Could you check a few things on this model? Use its own coordinates, in mm. Face numbers are marked on the shaded views. A direction names the side the tool comes from. Coordinates: 2 decimals unless noted, no trailing zeros. Loops run counter-clockwise (first coordinate to the right, second up) from the corner with the lowest first, then second, coordinate; pieces in that order, holes last. Notation, with made-up numbers: (57, 64) -> (90, 64) arc R21 cw to (90, 85) -> close; hole circle Ø10 at (57, -12). An arc over 180 degrees is marked (long way). One line per question, with ' | ' between items.
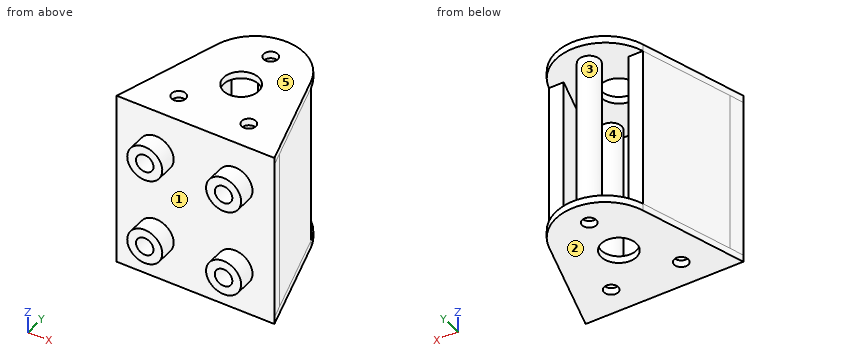
from build123d import *

# Parameters (mm, degrees)
SKETCH1_R           = 5
SKETCH1_R_2         = 2
BOSS_EXTRUDE1_DEPTH = 2
SKETCH2_R           = 2
SKETCH2_R_2         = 5
BOSS_EXTRUDE2_DEPTH = 2
SKETCH3_R           = 3
SKETCH3_R_2         = 2.5
BOSS_EXTRUDE3_DEPTH = 46
BOSS_EXTRUDE4_DEPTH = 46
BOSS_EXTRUDE5_DEPTH = 46
SKETCH8_R           = 5
SKETCH8_R_2         = 2.5
BOSS_EXTRUDE6_DEPTH = 5


with BuildPart() as part:
    # Sketch1 → Boss-Extrude1 (new body)
    with BuildSketch(Plane.XY):
        with BuildLine():
            Line((-22.5, 0), (22.5, 0))
            Line((22.5, 0), (13.399264765, 30.057056046))
            ThreePointArc((13.399264765, 30.057056046), (0, 40), (-13.399264765, 30.057056046))
            Line((-13.399264765, 30.057056046), (-22.5, 0))
        make_face()
        with Locations((0, 20)):
            Circle(SKETCH1_R, mode=Mode.SUBTRACT)
        with Locations((0, 33)):
            Circle(SKETCH1_R_2, mode=Mode.SUBTRACT)
        with Locations((10, 8)):
            Circle(SKETCH1_R_2, mode=Mode.SUBTRACT)
        with Locations((-10, 8)):
            Circle(SKETCH1_R_2, mode=Mode.SUBTRACT)
    extrude(amount=BOSS_EXTRUDE1_DEPTH)



with BuildPart() as body_2:
    # Sketch2 → Boss-Extrude2 (new body)
    with BuildSketch(Plane(origin=(0, 0, 50), x_dir=(-1, 0, 0), z_dir=(0, 0, -1))):
        with BuildLine():
            Line((-13.399264765, 30.057056046), (-22.5, 0))
            Line((-22.5, 0), (22.5, 0))
            Line((22.5, 0), (13.399264765, 30.057056046))
            ThreePointArc((13.399264765, 30.057056046), (0, 40), (-13.399264765, 30.057056046))
        make_face()
        with Locations(Location((-10, 8, 0), (0, 0, 180))):
            Circle(SKETCH2_R, mode=Mode.SUBTRACT)
        with Locations(Location((10, 8, 0), (0, 0, 180))):
            Circle(SKETCH2_R, mode=Mode.SUBTRACT)
        with Locations(Location((0, 20, 0), (0, 0, 180))):
            Circle(SKETCH2_R_2, mode=Mode.SUBTRACT)
        with Locations(Location((0, 33, 0), (0, 0, 180))):
            Circle(SKETCH2_R, mode=Mode.SUBTRACT)
    extrude(amount=BOSS_EXTRUDE2_DEPTH)


with BuildPart() as part_1:
    add(part.part)

    add(body_2.part)  # Boss-Extrude3 merges body 2
    # Sketch3 → Boss-Extrude3 (add)
    # profile 1 of 3: a face of its own
    with BuildSketch(Plane(origin=(0, 0, 48), x_dir=(-1, 0, 0), z_dir=(0, 0, -1))):
        with Locations(Location((10, 8, 0), (0, 0, 180))):
            Circle(SKETCH3_R)
        with Locations(Location((10, 8, 0), (0, 0, 180))):
            Circle(SKETCH3_R_2, mode=Mode.SUBTRACT)
    # profile 2 of 3: a face of its own
    with BuildSketch(Plane(origin=(0, 0, 48), x_dir=(-1, 0, 0), z_dir=(0, 0, -1))):
        with Locations(Location((0, 33, 0), (0, 0, 180))):
            Circle(SKETCH3_R)
        with Locations(Location((0, 33, 0), (0, 0, 180))):
            Circle(SKETCH3_R_2, mode=Mode.SUBTRACT)
    # profile 3 of 3: a face of its own
    with BuildSketch(Plane(origin=(0, 0, 48), x_dir=(-1, 0, 0), z_dir=(0, 0, -1))):
        with Locations(Location((-10, 8, 0), (0, 0, 180))):
            Circle(SKETCH3_R)
        with Locations(Location((-10, 8, 0), (0, 0, 180))):
            Circle(SKETCH3_R_2, mode=Mode.SUBTRACT)
    extrude(amount=BOSS_EXTRUDE3_DEPTH)

    # Sketch4 → Boss-Extrude4 (add)
    with BuildSketch(Plane(origin=(0, 0, 48), x_dir=(-1, 0, 0), z_dir=(0, 0, -1))):
        Polygon((22.5, 0), (-22.5, 0), (-21.288872041, 4), (21.288872041, 4), align=None)
    extrude(amount=BOSS_EXTRUDE4_DEPTH)

    # Sketch5 → Boss-Extrude5 (add)
    with BuildSketch(Plane(origin=(0, 0, 48), x_dir=(-1, 0, 0), z_dir=(0, 0, -1))):
        Polygon((17.109538251, 4), (21.288872041, 4), (13.399264765, 30.057056046), (9.219930974, 30.057056046), align=None)
        Polygon((-21.288872041, 4), (-17.109538251, 4), (-9.219930974, 30.057056046), (-13.399264765, 30.057056046), align=None)
    extrude(amount=BOSS_EXTRUDE5_DEPTH)

    # Sketch8 → Boss-Extrude6 (add)
    # profile 1 of 4: a face of its own
    with BuildSketch(Plane.XZ):
        with Locations(Location((-11.25, 12.5, 0), (0, 0, 90))):
            Circle(SKETCH8_R)
        with Locations(Location((-11.25, 12.5, 0), (0, 0, 270))):
            Circle(SKETCH8_R_2, mode=Mode.SUBTRACT)
    # profile 2 of 4: a face of its own
    with BuildSketch(Plane.XZ):
        with Locations(Location((-11.25, 37.5, 0), (0, 0, 90))):
            Circle(SKETCH8_R)
        with Locations(Location((-11.25, 37.5, 0), (0, 0, 90))):
            Circle(SKETCH8_R_2, mode=Mode.SUBTRACT)
    # profile 3 of 4: a face of its own
    with BuildSketch(Plane.XZ):
        with Locations(Location((11.25, 37.5, 0), (0, 0, 90))):
            Circle(SKETCH8_R)
        with Locations(Location((11.25, 37.5, 0), (0, 0, 270))):
            Circle(SKETCH8_R_2, mode=Mode.SUBTRACT)
    # profile 4 of 4: a face of its own
    with BuildSketch(Plane.XZ):
        with Locations(Location((11.25, 12.5, 0), (0, 0, 90))):
            Circle(SKETCH8_R)
        with Locations(Location((11.25, 12.5, 0), (0, 0, 90))):
            Circle(SKETCH8_R_2, mode=Mode.SUBTRACT)
    extrude(amount=BOSS_EXTRUDE6_DEPTH)


solid = part_1.part
1) If we section it at B-B on x = 0: Give the number of separate pieces and of enclosed holes in the cut face, and give its area (3 significant figures).
Data:
separate pieces: 3 | enclosed holes: 0 | area: 334 mm²
2) If we section it at A-A on z = 41.5: Please give me the cut outline in (x, y).
Data:
outline: (-22.5, 0) -> (-14.25, 0) -> (-14.25, -5) -> (-8.25, -5) -> (-8.25, 0) -> (8.25, 0) -> (8.25, -5) -> (14.25, -5) -> (14.25, 0) -> (22.5, 0) -> (13.4, 30.06) -> (9.22, 30.06) -> (17.11, 4) -> (-17.11, 4) -> (-9.22, 30.06) -> (-13.4, 30.06) -> close; circle Ø6 at (-10, 8); circle Ø6 at (0, 33); circle Ø6 at (10, 8); hole circle Ø5 at (-10, 8); hole circle Ø5 at (0, 33); hole circle Ø5 at (10, 8)
3) I'm going to push flat-ended pins straight in: pin 1 Ø1.5 at (x, z) = (13.5, 29) entering from -Y; pin 2 Ø4 at (y, z) = (31.5, 35.5) entering from -X; pin 3 Ø4 at (y, z) = (24.5, 12.5) entering from +X; pin 4 Ø2.5 at (x, y) = (10.5, 8.5) entering from +Z. Where does each tip first touch, or does it pass through?
Data:
pin 1: y = 0 | pin 2: x = -13.57 | pin 3: x = 15.69 | pin 4: through
4) If we section it at C-C on y = 12: Please give me the cut outline in (x, z).
Data:
outline: (-18.87, 0) -> (18.87, 0) -> (18.87, 50) -> (-18.87, 50) -> close; hole (-14.69, 2) -> (14.69, 2) -> (14.69, 48) -> (-14.69, 48) -> close
5) I need wall thicknesses on line 1 along Y through (x, z) = (0, 49); line 2 along Z through (x, y) = (11, -3); line 3 along Z through (x, y) = (-6.5, 7.5). Which ranges of each line are inside material? Lowest first, please. Write a range as from..to.
Data:
line 1: 0..15, 25..31, 35..40 | line 2: 7.51..10.01, 14.99..17.49, 32.51..35.01, 39.99..42.49 | line 3: 0..2, 48..50
6) On a 3-axis mill with a long thin cutter (end or side, diameter ignored), from which of +Z, -Z, +X, -X, +Y, -Y can I reach the whole of each face in a straight line? I mean the marked faces 4 and 5. Say none if no direction works.
Data:
face 4: none | face 5: +Z, +X, -X, +Y, -Y
7) We'd pull the mould along Y, two halves only. Please class the marked faces 1, 2 and 3: pulls with the +Y half, pulls with the -Y half, needs draft (parallel to the pull), parting line crosses it, or undercut.
Data:
face 1: pulls with the -Y half | face 2: needs draft | face 3: undercut
